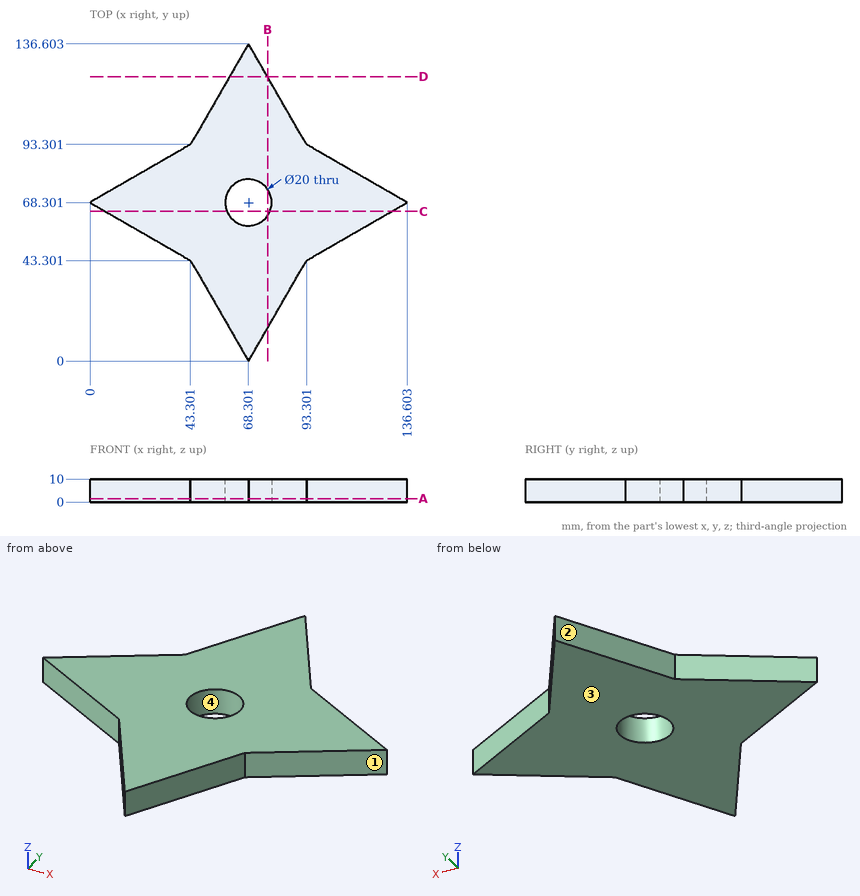
Geometry: see drawing. Coordinates: mm, zero at the bounding-box minimum. Give positions to 0.01 mm unless a question says otherwise; leave off trailing zeros. Write each loop counter-clockwise with the first axis right and the second up, starting at its lowest first coordinate (ties: lowest second). Pieces come first, ordered by that corner, then holes. Notation, with made-up numbers: M -13,-10 L 40,-10 A13 cw 40,9 Z; hole C 28,-36 d1. An arc over 180 degrees is marked long. Return JSON: item names as keys, results as strings. Group by question number.
1) Cut plane D-D, the plane y = 122.5. Output: boundary loops of the cut face in (x, z), then the cut area to 3 significant figures.
2) Draft query along X for the marked faces 1, 2, 3 and 4. Return one class per face: released by +X, released by -X, zero draft, split by the parting line, or undercut.
3) Cut plane C-C, the plane y = 64.5. Output: boundary loops of the cut face in (x, z).
4) Ray query, L1, parallel to X at y = 76, z = 0.75 (1 decimal); L2, parallel to X at y = 73, z = 6.25 (1 decimal). Return the intervals inside material, ascending.
5) Cut plane B-B, the plane x = 76.5. Output: boundary loops of the cut face in (y, z) (1 decimal).
6) Cut plane A-A, the plane z = 1.5. Output: boundary loops of the cut face in (x, y), then the cut area to 3 significant figures.
7) First-contact query: pin 1 Ø5 at (y, z) = (29, 5) entering from +X; pin 2 Ø4 at (x, z) = (14.5, 4) entering from -Y (1 decimal); pin 3 Ø4 at (x, z) = (121, 8.5) entering from +Y (1 decimal). Flat tips, straight axial feed; report the tip coordinate or a pass-through.
Data:
{
 "1": {"outline": "M 60.16,0 L 76.44,0 L 76.44,10 L 60.16,10 Z", "area": "163 mm²"},
 "2": {"face 1": "released by +X", "face 2": "released by -X", "face 3": "zero draft", "face 4": "undercut"},
 "3": {"outline": "M 6.58,0 L 59.05,0 L 59.05,10 L 6.58,10 Z; M 77.55,0 L 130.02,0 L 130.02,10 L 77.55,10 Z"},
 "4": {"L1": "x = 13.3 to 61.9, 74.7 to 123.3", "L2": "x = 8.1 to 59.5, 77.1 to 128.5"},
 "5": {"outline": "M 14.2,0 L 62.6,0 L 62.6,10 L 14.2,10 Z; M 74,0 L 122.4,0 L 122.4,10 L 74,10 Z"},
 "6": {"outline": "M 0,68.3 L 43.3,43.3 L 68.3,0 L 93.3,43.3 L 136.6,68.3 L 93.3,93.3 L 68.3,136.6 L 43.3,93.3 Z; hole C 68.3,68.3 d20", "area": "6,520 mm²"},
 "7": {"pin 1": "stops at x = 86.49", "pin 2": "stops at y = 58.8", "pin 3": "stops at y = 78.5"}
}
